from build123d import *
from build123d.topology import SkipClean

# Parameters (mm, degrees)
SKETCH1_W           = 60
SKETCH1_H           = 49
SKETCH1_R           = 2
SKETCH1_W_2         = 46
SKETCH1_H_2         = 35
BOSS_EXTRUDE1_DEPTH = 10
SKETCH6_R           = 2
CUT_EXTRUDE3_DEPTH  = 50.244289182
SKETCH7_W           = 7
SKETCH7_H           = 7
SKETCH7_R           = 2
BOSS_EXTRUDE4_DEPTH = 25
SKETCH10_R          = 25
SKETCH10_R_2        = 20
BOSS_EXTRUDE5_DEPTH = 25
FILLET2_R           = 3


with BuildPart() as part:
    # Sketch1 → Boss-Extrude1 (new body)
    with BuildSketch(Plane(origin=(0, 0, 0), x_dir=(1, 0, 0), z_dir=(0, 1, 0))):
        Rectangle(SKETCH1_W, SKETCH1_H)
        with Locations(Location((-26, 20.5, 0), (0, 0, 270))):
            Circle(SKETCH1_R, mode=Mode.SUBTRACT)
        with Locations(Location((26, 20.5, 0), (0, 0, 90))):
            Circle(SKETCH1_R, mode=Mode.SUBTRACT)
        with Locations(Location((26, -20.5, 0), (0, 0, 270))):
            Circle(SKETCH1_R, mode=Mode.SUBTRACT)
        with Locations(Location((-26, -20.5, 0), (0, 0, 90))):
            Circle(SKETCH1_R, mode=Mode.SUBTRACT)
        Rectangle(SKETCH1_W_2, SKETCH1_H_2, mode=Mode.SUBTRACT)
    extrude(amount=BOSS_EXTRUDE1_DEPTH)

    # Sketch9 → Loft1 section 0
    with BuildSketch(Plane(origin=(0, 10, 0), x_dir=(1, 0, 0), z_dir=(0, 1, 0))):
        with BuildLine():
            Line((30, -24.5), (-30, -24.5))
            Line((-30, -24.5), (-30, 24.5))
            Line((-30, 24.5), (30, 24.5))
            Line((30, 24.5), (30, -24.5))
        make_face()
    # Sketch8 for Loft1 → Loft1 section 1
    with BuildSketch(Plane(origin=(0, 30, 0), x_dir=(1, 0, 0), z_dir=(0, 1, 0))):
        with BuildLine():
            # circular arc as an exact rational Bezier (weights 1, cos(half-angle), 1)
            Bezier((19.36330319, -15.813364272), (0, -39.523531441), (-19.36330319, -15.813364272), weights=[1, 0.632534571, 1])
            Bezier((-19.36330319, -15.813364272), (-32.277550677, 0), (-19.36330319, 15.813364272), weights=[1, 0.774532128, 1])
            Bezier((-19.36330319, 15.813364272), (0, 39.523531441), (19.36330319, 15.813364272), weights=[1, 0.632534571, 1])
            Bezier((19.36330319, 15.813364272), (32.277550677, 0), (19.36330319, -15.813364272), weights=[1, 0.774532128, 1])
        make_face()
    loft()

    # Sketch2 → Cut-Loft1 section 0
    with BuildSketch(Plane(origin=(0, 10, 0), x_dir=(1, 0, 0), z_dir=(0, 1, 0))):
        with BuildLine():
            Line((-23, -17.5), (23, -17.5))
            Line((23, -17.5), (23, 17.5))
            Line((23, 17.5), (-23, 17.5))
            Line((-23, 17.5), (-23, -17.5))
        make_face()
    # Sketch3 for Cut-Loft1 → Cut-Loft1 section 1
    with BuildSketch(Plane(origin=(0, 30, 0), x_dir=(1, 0, 0), z_dir=(0, 1, 0))):
        with BuildLine():
            Bezier((-15.916573882, -12.11043665), (0, -33.029362323), (15.916573882, -12.11043665), weights=[1, 0.605521832, 1])
            Bezier((15.916573882, -12.11043665), (25.131036551, 0), (15.916573882, 12.11043665), weights=[1, 0.795828694, 1])
            Bezier((15.916573882, 12.11043665), (0, 33.029362323), (-15.916573882, 12.11043665), weights=[1, 0.605521832, 1])
            Bezier((-15.916573882, 12.11043665), (-25.131036551, 0), (-15.916573882, -12.11043665), weights=[1, 0.795828694, 1])
        make_face()
    loft(mode=Mode.SUBTRACT)

    # Sketch6 → Cut-Extrude3 (cut, through all)
    with SkipClean():  # the faces are left unmerged after this step: merging them gives an invalid solid
        with BuildSketch(Plane.XZ):
            with Locations(Location((26, 20.5, 0), (0, 0, 202.73857606))):
                Circle(SKETCH6_R)
            with Locations(Location((26, -20.5, 0), (0, 0, 270))):
                Circle(SKETCH6_R)
            with Locations(Location((-26, -20.5, 0), (0, 0, 235.736158167))):
                Circle(SKETCH6_R)
            with Locations(Location((-26, 20.5, 0), (0, 0, 270))):
                Circle(SKETCH6_R)
        extrude(amount=-CUT_EXTRUDE3_DEPTH, mode=Mode.SUBTRACT)

    # Sketch7 → Boss-Extrude4 (add)
    # profile 1 of 4: a face of its own
    with BuildSketch(Plane.XZ):
        with Locations((-26.5, 21)):
            Rectangle(SKETCH7_W, SKETCH7_H)
        with Locations(Location((-26, 20.5, 0), (0, 0, 270))):
            Circle(SKETCH7_R, mode=Mode.SUBTRACT)
    # profile 2 of 4: a face of its own
    with BuildSketch(Plane.XZ):
        with Locations((-26.5, -21)):
            Rectangle(SKETCH7_W, SKETCH7_H)
        with Locations(Location((-26, -20.5, 0), (0, 0, 90))):
            Circle(SKETCH7_R, mode=Mode.SUBTRACT)
    # profile 3 of 4: a face of its own
    with BuildSketch(Plane.XZ):
        with Locations((26.5, -21)):
            Rectangle(SKETCH7_W, SKETCH7_H)
        with Locations(Location((26, -20.5, 0), (0, 0, 270))):
            Circle(SKETCH7_R, mode=Mode.SUBTRACT)
    # profile 4 of 4: a face of its own
    with BuildSketch(Plane.XZ):
        with Locations((26.5, 21)):
            Rectangle(SKETCH7_W, SKETCH7_H)
        with Locations(Location((26, 20.5, 0), (0, 0, 90))):
            Circle(SKETCH7_R, mode=Mode.SUBTRACT)
    extrude(amount=-BOSS_EXTRUDE4_DEPTH)


with BuildPart() as boss_extrude5_tool:
    # Sketch10 → Boss-Extrude5 (new body)
    with BuildSketch(Plane(origin=(0, 30, 0), x_dir=(1, 0, 0), z_dir=(0, 1, 0))):
        with Locations(Location((0, 0, 0), (0, 0, 140.762632884))):
            Circle(SKETCH10_R)
        with Locations(Location((0, 0, 0), (0, 0, 37.266416314))):
            Circle(SKETCH10_R_2, mode=Mode.SUBTRACT)
    extrude(amount=BOSS_EXTRUDE5_DEPTH)


with BuildPart() as part_1:
    add(part.part)


with BuildPart() as part_2:
    # Boss-Extrude5: joined with boss_extrude5_tool
    add(part_1.part.fuse(boss_extrude5_tool.part, tol=0.00001))

    # Fillet2
    fillet2_edges = [part_2.edges().sort_by_distance(p)[0] for p in [
        (30, 12.5, 24.5),
        (-30, 12.5, 24.5),
        (-30, 12.5, -24.5),
        (30, 12.5, -24.5),
    ]]
    fillet(fillet2_edges, radius=FILLET2_R)


solid = part_2.part
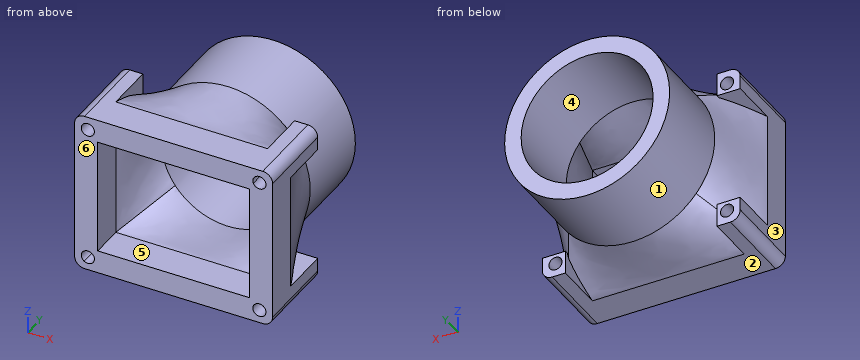
Model file for the job. Use its own axes, mm. Face numbers are marked on the shaded views. A direction names the side the tool comes from. Give positions to 0.01 mm unless a question says otherwise; leave off trailing zeros. Loops run counter-clockwise (first coordinate to the right, second up) from the corner with the lowest first, then second, coordinate; pieces in that order, holes last. Notation, with made-up numbers: (70.5, 61) -> (93.5, 61) arc R22 ccw to (93.5, 74) -> close; hole circle Ø8 at (-19.75, -37.5). An arc over 180 degrees is marked (long way). Use a Markdown table: item, result. Add a question column.
(1) Slice it at A-A on y = 4. List the corners of the cut face in (x, z).
(2) Wall check: line 1 along Z through (x, y) = (-26, 2.75); line 2 along X through (y, z) = (7.25, -20.5); line 3 along X through (y, z) = (22, 20). Give the ranges that are in metal, low to high.
(3) Drop flat-ended pins along their axis: pin 1 Ø7.5 at (x, y) = (-25.5, 19) entering from +Z; pin 2 Ø3.5 at (x, z) = (26, 20.5) entering from -Y; pin 3 Ø5 at (x, z) = (-26, -20.5) entering from +Y; pin 4 Ø4 at (x, y) = (-20.5, 31) entering from -Z. Give the stop position or say it passes through.
(4) Mould opens along Z. For the marked faces 1, 2, 3 and 4 say: +Z half, -Z half, draft (parallel to the pull), parting line (faces both ways), or undercut.
(5) Tool access for the marked faces 5 and 6: list every direction of +Z, -Z, +X, -X, +Y, -Y with a clear straight run to the whole face (end or side of a thin tool).
Filled sheet:
| question | item | result |
|---|---|---|
| 1 | outline | (-30, -21.5) arc R3 ccw to (-27, -24.5) -> (27, -24.5) arc R3 ccw to (30, -21.5) -> (30, 21.5) arc R3 ccw to (27, 24.5) -> (-27, 24.5) arc R3 ccw to (-30, 21.5) -> close; hole circle Ø4 at (-26, -20.5); hole circle Ø4 at (-26, 20.5); hole (-23, -17.5) -> (23, -17.5) -> (23, 17.5) -> (-23, 17.5) -> close; hole circle Ø4 at (26, -20.5); hole circle Ø4 at (26, 20.5) |
| 2 | line 1 | -24.5 to -22.5, -18.5 to 18.5, 22.5 to 24.5 |
| 2 | line 2 | -30 to -28, -24 to 24, 28 to 30 |
| 2 | line 3 | -30 to -27.94, -24.06 to -23, -22.04 to 22.04, 23 to 24.06, 27.94 to 30 |
| 3 | pin 1 | z = 24.5 |
| 3 | pin 2 | through |
| 3 | pin 3 | y = 25 |
| 3 | pin 4 | z = -16.82 |
| 4 | face 1 | parting line |
| 4 | face 2 | -Z half |
| 4 | face 3 | draft |
| 4 | face 4 | undercut |
| 5 | face 5 | -Y |
| 5 | face 6 | +Z, -Z, +X, -X, -Y |
